Input: part model. Units: mm. Frame: model coordinates. Face numbers are marked on the shaded views. A direction names the side the tool comes from. Round coordinates to 2 decimals unless told otherwise and drop trailing zeros. Write each loop counter-clockwise with the first axis right and the second up, starting at its lowest first coordinate (ties: lowest second). Pieces come first, ordered by that corner, then holes. Notation, with made-up numbers: (48.25, 53) -> (97.25, 53) arc R18 cw to (97.25, 77) -> close; hole circle Ø5 at (-12.75, 76). An arc over 180 degrees is marked (long way). Use CSV: the item, a comma, the result in double quotes.
```python
from build123d import *

# Parameters (mm, degrees)
SKETCH1_R           = 15.875
BOSS_EXTRUDE1_DEPTH = 50.8
SKETCH2_W           = 31.75
SKETCH2_H           = 50.8
BOSS_EXTRUDE2_DEPTH = 4.7625
SKETCH3_W           = 88.9
SKETCH3_H           = 41.148
BOSS_EXTRUDE3_DEPTH = 41.2496
CUT_EXTRUDE2_DEPTH  = 111.191148756


with BuildPart() as part:
    # Sketch1 → Boss-Extrude1 (new body)
    with BuildSketch(Plane.XY):
        Circle(SKETCH1_R)
    extrude(amount=BOSS_EXTRUDE1_DEPTH)

    # Sketch2 → Boss-Extrude2 (add)
    with BuildSketch(Plane(origin=(0, 0, 0), x_dir=(-1, 0, 0), z_dir=(0, 0, -1))):
        with Locations((0, 25.4)):
            Rectangle(SKETCH2_W, SKETCH2_H)
    extrude(amount=-BOSS_EXTRUDE2_DEPTH)

    # Sketch3 → Boss-Extrude3 (add)
    with BuildSketch(Plane(origin=(0, 50.8, 0), x_dir=(1, 0, 0), z_dir=(0, 1, 0))):
        with Locations((0, -2.38125)):
            Rectangle(SKETCH3_W, SKETCH3_H)
    extrude(amount=BOSS_EXTRUDE3_DEPTH)

    # Sketch5 → Cut-Extrude2 (cut, through all)
    with BuildSketch(Plane.XY.offset(22.95525)):
        Polygon((-6.3246, 92.0496), (-6.3246, 90.297), (-31.70428, 90.297), (-31.70428, 52.2224), (31.70428, 52.2224), (31.70428, 90.297), (6.3246, 90.297), (6.3246, 92.0496), align=None)
    extrude(amount=-CUT_EXTRUDE2_DEPTH, mode=Mode.SUBTRACT)


solid = part.part
```
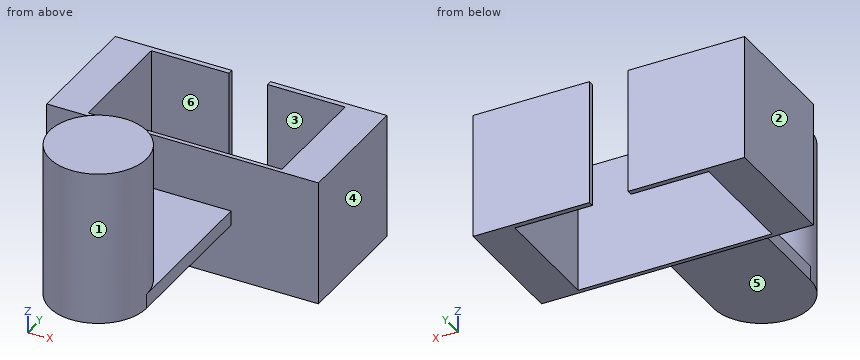
Item 1: Section query D-D on x = 0. Return the cut outline in (y, z) (1 decimal).
Worked answers:
outline,"(-15.9, 0) -> (50.8, 0) -> (50.8, -18.2) -> (52.2, -18.2) -> (52.2, 23) -> (50.8, 23) -> (50.8, 4.8) -> (15.9, 4.8) -> (15.9, 50.8) -> (-15.9, 50.8) -> close"
Item 2: Section query B-B on x = -22. Return the cut outline in (y, z).
Worked answers:
outline,"(50.8, -18.19) -> (52.22, -18.19) -> (52.22, 22.96) -> (50.8, 22.96) -> close; (90.3, -18.19) -> (92.05, -18.19) -> (92.05, 22.96) -> (90.3, 22.96) -> close"
Item 3: Line query: line 1 (Y direction, x = -19.5, z = 20); line 2 (X direction, y = 55, z = -10); line 3 (Z direction, x = -2.5, y = 1). Output: solid intervals per line, ascending.
Worked answers:
line 1,"y = 50.8 to 52.22, 90.3 to 92.05"
line 2,"x = -44.45 to -31.7, 31.7 to 44.45"
line 3,"z = 0 to 50.8"
Item 4: Set-up query: the marked faces 1, 2 and 3. Return all of +Z, -Z, +X, -X, +Y, -Y with unobstructed straight access to the full face (end or side cutting, diameter ignored); none if empty.
Worked answers:
face 1,"+Z"
face 2,"+Z, -Z, -X, +Y, -Y"
face 3,"+Z, -Z"
Item 5: First-contact query: pin 1 Ø9.5 at (x, y) = (-7, 22) entering from -Z; pin 2 Ø1.4 at (y, z) = (14.5, 1.5) entering from +X (3 decimals); pin 3 Ø20.5 at (x, z) = (7.5, 4) entering from -Y (3 decimals); pin 4 Ø2.5 at (y, z) = (13.5, 1.5) entering from -X (3 decimals). Flat tips, straight axial feed; report the tip coordinate or a pass-through.
Worked answers:
pin 1,"stops at z = 0"
pin 2,"stops at x = 15.875"
pin 3,"stops at y = -15.875"
pin 4,"stops at x = -15.875"
Item 6: Section query C-C on z = -6. Return the cut outline in (x, y), plus the area to 3 significant figures.
Worked answers:
outline,"(-44.45, 50.8) -> (44.45, 50.8) -> (44.45, 92.05) -> (6.32, 92.05) -> (6.32, 90.3) -> (31.7, 90.3) -> (31.7, 52.22) -> (-31.7, 52.22) -> (-31.7, 90.3) -> (-6.32, 90.3) -> (-6.32, 92.05) -> (-44.45, 92.05) -> close"
area,"1,230 mm²"
Item 7: Section query A-A on y = 82.5. Return the cut outline in (x, z).
Worked answers:
outline,"(-44.45, -18.19) -> (-31.7, -18.19) -> (-31.7, 22.96) -> (-44.45, 22.96) -> close; (31.7, -18.19) -> (44.45, -18.19) -> (44.45, 22.96) -> (31.7, 22.96) -> close"
Item 8: Pull-direction query (X, two-part tool) for the marked faces 4, 5 and 6; classes: +X half, -X half, draft (parallel to the pull), parting line (faces both ways), or undercut.
Worked answers:
face 4,"+X half"
face 5,"draft"
face 6,"undercut"
